Here's how the part is built. I have some questions about the finished solid (model axes, mm). Face numbers are marked on the shaded views. A direction names the side the tool comes from. Round coordinates to 2 decimals unless told otherwise and drop trailing zeros. Loops run counter-clockwise (first coordinate to the right, second up) from the corner with the lowest first, then second, coordinate; pieces in that order, holes last. Notation, with made-up numbers: M 2,22 L 26,22 A5 cw 26,27 Z; hole C -0.5,43.5 d1. An arc over 180 degrees is marked long. Use a Markdown table: item, result.
from build123d import *

# Parameters (mm, degrees)
BOSS_EXTRUDE1_DEPTH = 1
BOSS_EXTRUDE2_DEPTH = 7.95
BOSS_EXTRUDE3_DEPTH = 16.45
SKETCH5_W           = 7.62
SKETCH5_H           = 2.54
SKETCH5_W_2         = 1.768524962
SKETCH5_H_2         = 1.697224475
BOSS_EXTRUDE4_DEPTH = 7.62
SKETCH6_R           = 2.95
BOSS_EXTRUDE5_DEPTH = 4


with BuildPart() as part:
    # Sketch1 → Boss-Extrude1 (new body)
    with BuildSketch(Plane(origin=(0, 0, 0), x_dir=(1, 0, 0), z_dir=(0, 1, 0))):
        with BuildLine():
            ThreePointArc((-27, -7.56), (-26.256051224, -9.356051224), (-24.46, -10.1))
            Line((-24.46, -10.1), (24.46, -10.1))
            ThreePointArc((24.46, -10.1), (26.256051224, -9.356051224), (27, -7.56))
            Line((27, -7.56), (27, -7))
            Line((27, -7), (24, -7))
            ThreePointArc((24, -7), (22, -5), (24, -3))
            Line((24, -3), (27, -3))
            Line((27, -3), (27, 3))
            Line((27, 3), (24, 3))
            ThreePointArc((24, 3), (22, 5), (24, 7))
            Line((24, 7), (27, 7))
            Line((27, 7), (27, 7.56))
            ThreePointArc((27, 7.56), (26.256051224, 9.356051224), (24.46, 10.1))
            Line((24.46, 10.1), (-24.46, 10.1))
            ThreePointArc((-24.46, 10.1), (-26.256051224, 9.356051224), (-27, 7.56))
            Line((-27, 7.56), (-27, 7))
            Line((-27, 7), (-24, 7))
            ThreePointArc((-24, 7), (-22, 5), (-24, 3))
            Line((-24, 3), (-27, 3))
            Line((-27, 3), (-27, -3))
            Line((-27, -3), (-24, -3))
            ThreePointArc((-24, -3), (-22, -5), (-24, -7))
            Line((-24, -7), (-27, -7))
            Line((-27, -7), (-27, -7.56))
        make_face()
    extrude(amount=BOSS_EXTRUDE1_DEPTH)

    # Sketch3 → Boss-Extrude2 (add)
    with BuildSketch(Plane(origin=(0, 1, 0), x_dir=(1, 0, 0), z_dir=(0, 1, 0))):
        with BuildLine():
            Line((-17.86, -10.1), (17.86, -10.1))
            ThreePointArc((17.86, -10.1), (19.656051224, -9.356051224), (20.4, -7.56))
            Line((20.4, -7.56), (20.4, 7.56))
            ThreePointArc((20.4, 7.56), (19.656051224, 9.356051224), (17.86, 10.1))
            Line((17.86, 10.1), (-17.86, 10.1))
            ThreePointArc((-17.86, 10.1), (-19.656051224, 9.356051224), (-20.4, 7.56))
            Line((-20.4, 7.56), (-20.4, -7.56))
            ThreePointArc((-20.4, -7.56), (-19.656051224, -9.356051224), (-17.86, -10.1))
        make_face()
    extrude(amount=BOSS_EXTRUDE2_DEPTH)

    # Sketch4 → Boss-Extrude3 (add)
    with BuildSketch(Plane.XZ):
        with BuildLine():
            Line((-17.86, -10.1), (17.86, -10.1))
            ThreePointArc((17.86, -10.1), (19.656051224, -9.356051224), (20.4, -7.56))
            Line((20.4, -7.56), (20.4, 7.56))
            ThreePointArc((20.4, 7.56), (19.656051224, 9.356051224), (17.86, 10.1))
            Line((17.86, 10.1), (-17.86, 10.1))
            ThreePointArc((-17.86, 10.1), (-19.656051224, 9.356051224), (-20.4, 7.56))
            Line((-20.4, 7.56), (-20.4, -7.56))
            ThreePointArc((-20.4, -7.56), (-19.656051224, -9.356051224), (-17.86, -10.1))
        make_face()
    extrude(amount=BOSS_EXTRUDE3_DEPTH)

    # Sketch5 → Boss-Extrude4 (add)
    with BuildSketch(Plane.ZY.offset(20.4)):
        with Locations((0, -10.377289394)):
            Rectangle(SKETCH5_W, SKETCH5_H)
        with Locations((0, -10.377289394)):
            Rectangle(SKETCH5_W_2, SKETCH5_H_2, mode=Mode.SUBTRACT)
        with Locations((-2.54, -10.377289394)):
            Rectangle(SKETCH5_W_2, SKETCH5_H_2, mode=Mode.SUBTRACT)
        with Locations((2.54, -10.377289394)):
            Rectangle(SKETCH5_W_2, SKETCH5_H_2, mode=Mode.SUBTRACT)
    extrude(amount=BOSS_EXTRUDE4_DEPTH)

    # Sketch6 → Boss-Extrude5 (add)
    with BuildSketch(Plane(origin=(0, 8.95, 0), x_dir=(1, 0, 0), z_dir=(0, 1, 0))):
        with Locations((-12.7, 0)):
            Circle(SKETCH6_R)
    extrude(amount=BOSS_EXTRUDE5_DEPTH)


solid = part.part
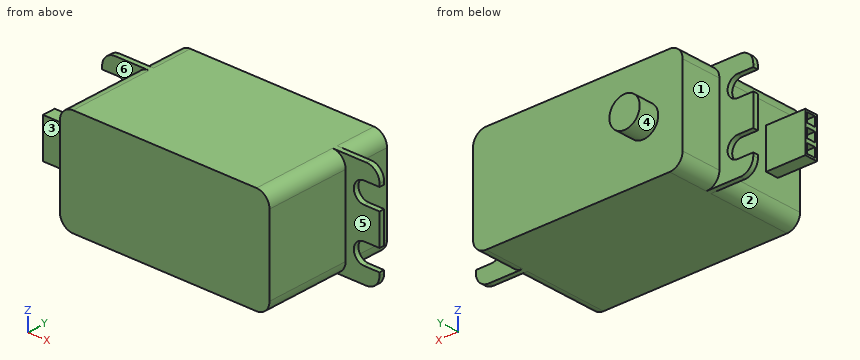
1. Imagine slicing it at C-C, the plane z = 5. Write out the boundary of the cut face in (x, y), then the cut area to 3 significant figures.
Answer sheet:
| item | result |
|---|---|
| outline | M -22,0 L -20.4,0 L -20.4,-16.45 L 20.4,-16.45 L 20.4,0 L 22,0 L 22,1 L 20.4,1 L 20.4,8.95 L -20.4,8.95 L -20.4,1 L -22,1 Z |
| area | 1,040 mm2 |
2. We'd pull the mould along Y, two halves only. Please class the marked faces 4, 5 and 6: +Y half, -Y half, draft (parallel to the pull), parting line (faces both ways), or undercut.
Answer sheet:
| item | result |
|---|---|
| face 4 | draft |
| face 5 | -Y half |
| face 6 | undercut |
3. Which directions (+Z, -Z, +X, -X, +Y, -Y) give clear straight access to the entire face, cutting with the end or side of a thin tool? Please do the marked faces 1, 2 and 3.
Answer sheet:
| item | result |
|---|---|
| face 1 | +Z, -Z, -X, +Y |
| face 2 | -Z, -X, -Y |
| face 3 | +Z, -Z, -X, -Y |
4. For pin 1 Ø5 at (y, z) = (-6, 0.5) entering from +X; pin 2 Ø0.5 at (x, y) = (-25.5, 0.5) entering from -Z; pin 3 Ø1 at (y, z) = (8, -7.5) entering from -X, each with a flat end and sliding along its axis, tell me the tip position at first contact or that it passes through.
Answer sheet:
| item | result |
|---|---|
| pin 1 | x = 20.4 |
| pin 2 | z = -9.97 |
| pin 3 | x = -20.4 |
5. Imagine slicing it at D-D, the plane z = -5.5. Write out the boundary of the cut face in (x, y).
Answer sheet:
| item | result |
|---|---|
| outline | M -22.06,0 L -20.4,0 L -20.4,-16.45 L 20.4,-16.45 L 20.4,0 L 22.06,0 L 22.06,1 L 20.4,1 L 20.4,8.95 L -20.4,8.95 L -20.4,1 L -22.06,1 Z |
6. Imagine slicing it at B-B, the plane x = -12.7. Write out the boundary of the cut face in (y, z), then the cut area to 3 significant figures.
Answer sheet:
| item | result |
|---|---|
| outline | M -16.45,-10.1 L 8.95,-10.1 L 8.95,-2.95 L 12.95,-2.95 L 12.95,2.95 L 8.95,2.95 L 8.95,10.1 L -16.45,10.1 Z |
| area | 537 mm2 |
7. Imagine slicing it at A-A, the plane y = -2.5. Write out the boundary of the cut face in (x, z).
Answer sheet:
| item | result |
|---|---|
| outline | M -20.4,-7.56 A2.54 ccw -17.86,-10.1 L 17.86,-10.1 A2.54 ccw 20.4,-7.56 L 20.4,7.56 A2.54 ccw 17.86,10.1 L -17.86,10.1 A2.54 ccw -20.4,7.56 Z |
8. I need wall thicknesses on probe 1 along Y at (x, z) = (-24.5, 0); probe 2 along Y at (x, z) = (10.5, -4.5); probe 3 along X at (y, z) = (6.5, 1.5). Which ranges of each line are inside material? Lowest first, please. Write a range as from..to.
Answer sheet:
| item | result |
|---|---|
| probe 1 | -11.65..-11.23, -9.53..-9.11, 0..1 |
| probe 2 | -16.45..8.95 |
| probe 3 | -20.4..20.4 |
